Autodesk Inventor part; units mm, degrees
ref_plane "YZ Plane" through (0, 0, 0) normal (1, 0, 0) x (0, 1, 0)
ref_plane "XZ Plane" through (0, 0, 0) normal (0, 1, 0) x (-1, 0, 0)
ref_plane "XY Plane" through (0, 0, 0) normal (0, 0, 1) x (1, 0, 0)
sketch "Sketch2" plane through (0, 0, 0) normal (0, 1, 0) x (-1, 0, 0)
  line L0 (-60, 70) -> (60, 70)
  line L1 (60, -70) -> (-60, -70)
  line L2 (-60, 70) -> (60, -70) construction
  line L3 (60, 70) -> (-60, -70) construction
  line L4 (-60, 55) -> (-30, 55)
  line L5 (-30, 55) -> (-30, -15)
  line L6 (-30, -15) -> (-60, -15)
  line L7 (-60, -15) -> (-60, 55)
  line L8 (60, 55) -> (30, 55)
  line L9 (30, 55) -> (30, -13)
  line L10 (30, -13) -> (60, -13)
  line L11 (60, 70) -> (60, 55)
  line L12 (60, -13) -> (60, -70)
  line L13 (-60, -70) -> (-60, -15)
  line L14 (-60, 55) -> (-60, 70)
  point P0 (0, 0)
  dimension "d9" = 120
  dimension "d10" = 140
  dimension "d11" = 30
  dimension "d12" = 70
  dimension "d13" = 15
  dimension "d17" = 68
  dimension "d18" = 15
extrude "Extrusion2" add sketch "Sketch2" along normal blind 3 contours L0 L11 L8 L9 L10 L12 L1 L13 L6 L5 L4 L14
properties part number "base"
Geometry check sheet. Reference: the model listing, model coordinates, mm. A direction names the side the tool comes from. Give positions to 0.01 mm unless a question says otherwise; leave off trailing zeros. Loops run counter-clockwise (first coordinate to the right, second up) from the corner with the lowest first, then second, coordinate; pieces in that order, holes last. Notation, with made-up numbers: M 79.5,7.25 L 98.5,7.25 A21 ccw 98.5,26.25 Z; hole C 57,42.25 d11. An arc over 180 degrees is marked long. Write each question's results on one line, items separated by ' | '.
1) Section check C-C, the plane z = 36.5. Record the boundary of the cut face in (x, y), plus the area to 3 significant figures.
Answers follow:
outline: M -30,0 L 30,0 L 30,3 L -30,3 Z | area: 180 mm2
2) Section check B-B, the plane y = 0.85. Record the boundary of the cut face in (x, z), plus the area to 3 significant figures.
Answers follow:
outline: M -60,-70 L 60,-70 L 60,-15 L 30,-15 L 30,55 L 60,55 L 60,70 L -60,70 L -60,55 L -30,55 L -30,-13 L -60,-13 Z | area: 12,700 mm2
3) Thickness scan on line 1 (Z direction, x = -32.5, y = 2.7); line 2 (Z direction, x = 53, y = 1.05); line 3 (X direction, y = 1.85, z = -14). Record the ranges inside material, lowest first.
Answers follow:
line 1: -70 to -13, 55 to 70 | line 2: -70 to -15, 55 to 70 | line 3: -60 to 30
4) Gauge pin test, flat end, axial feed: pin 1 (1.5 mm diameter, centred on y = 1.5, z = 9, fed in from -X). Record the tip position at first contact, or that the pin passes through.
Answers follow:
pin 1: x = -30
5) Tool access check on faces 1 (the face through (30, 1, 20)), 2 (the face through (1, 3, 1)), 3 (the face through (-45, 1, -13)). Record the directions out of +Z, -Z, +X, -X, +Y, -Y that give a thin tool (end or side, any length) a straight path to the whole face; none if there is none.
Answers follow:
face 1: +X, +Y, -Y | face 2: +Z, -Z, +X, -X, +Y | face 3: -X, +Y, -Y
6) Section check A-A, the plane x = 35. Record the boundary of the cut face in (y, z), plus the area to 3 significant figures.
Answers follow:
outline: M 0,-70 L 3,-70 L 3,-15 L 0,-15 Z; M 0,55 L 3,55 L 3,70 L 0,70 Z | area: 210 mm2
7) Release check for a two-part mould opening along Z. For faces 4 (the face through (-45, 1, 55)), 5 (the face through (1, 1, 70)), 6 (the face through (-60, 1, 63)), 7 (the face through (-1, 1, -70)) record: +Z half, -Z half, draft (parallel to the pull), parting line (faces both ways), or undercut.
Answers follow:
face 4: undercut | face 5: +Z half | face 6: draft | face 7: -Z half
